from build123d import *

# Parameters (mm, degrees)
F0_W      = 43.942
F0_H      = 2.159
F0_W_2    = 6.858
F1_DEPTH  = 25.4
F0_R      = 2.159
F2_DEPTH  = 3.175
F3_R      = 2.159
F4_DEPTH  = 3.175
F6_R      = 2.159
F7_DEPTH  = 3.175
F9_R      = 2.159
F10_DEPTH = 3.175


with BuildPart() as f1:
    # F0 (on Right) → F1 (new body)
    with BuildSketch(Plane.YZ):
        with Locations((-17.288983049, 3.5224220661)):
            Rectangle(F0_W, F0_H)
        with Locations((8.111016951, 3.5224220661)):
            Rectangle(F0_W_2, F0_H)
    extrude(amount=F1_DEPTH)

    # F0 (on Right) → F2 (join)
    with BuildSketch(Plane.YZ):
        with BuildLine():
            Line((4.682016951, 8.5389220661), (4.682016951, 4.6019220661))
            Line((4.682016951, 4.6019220661), (11.540016951, 4.6019220661))
            Line((11.540016951, 4.6019220661), (11.540016951, 8.5389220661))
            ThreePointArc((11.540016951, 8.5389220661), (8.111016951, 5.1099220661), (4.682016951, 8.5389220661))
        make_face()
        with BuildLine():
            ThreePointArc((11.540016951, 8.5389220661), (8.111016951, 11.9679220661), (4.682016951, 8.5389220661))
            ThreePointArc((4.682016951, 8.5389220661), (8.111016951, 5.1099220661), (11.540016951, 8.5389220661))
        make_face()
        with Locations((8.111016951, 8.5389220661)):
            Circle(F0_R, mode=Mode.SUBTRACT)
    extrude(amount=F2_DEPTH)

    # F3 (on face) → F4 (join)
    with BuildSketch(Plane.YZ.offset(25.4)):
        with BuildLine():
            ThreePointArc((4.682016951, 8.5389220661), (8.111016951, 5.1099220661), (11.540016951, 8.5389220661))
            ThreePointArc((11.540016951, 8.5389220661), (8.111016951, 11.9679220661), (4.682016951, 8.5389220661))
        make_face()
        with Locations((8.111016951, 8.5389220661)):
            Circle(F3_R, mode=Mode.SUBTRACT)
        with BuildLine():
            Line((11.540016951, 4.6019220661), (11.540016951, 8.5389220661))
            ThreePointArc((11.540016951, 8.5389220661), (8.111016951, 5.1099220661), (4.682016951, 8.5389220661))
            Line((4.682016951, 8.5389220661), (4.682016951, 4.6019220661))
            Line((4.682016951, 4.6019220661), (11.540016951, 4.6019220661))
        make_face()
    extrude(amount=-F4_DEPTH)

    # F6 (on offset) → F7 (join)
    with BuildSketch(Plane.YZ.offset(7.112)):
        with BuildLine():
            Line((11.540016951, 4.6019220661), (11.540016951, 8.5389220661))
            ThreePointArc((11.540016951, 8.5389220661), (8.111016951, 11.9679220661), (4.682016951, 8.5389220661))
            Line((4.682016951, 8.5389220661), (4.682016951, 4.6019220661))
            Line((4.682016951, 4.6019220661), (11.540016951, 4.6019220661))
        make_face()
        with Locations((8.111016951, 8.5389220661)):
            Circle(F6_R, mode=Mode.SUBTRACT)
    extrude(amount=F7_DEPTH)

    # F9 (on offset) → F10 (join)
    with BuildSketch(Plane.YZ.offset(18.288)):
        with BuildLine():
            Line((4.682016951, 8.5389220661), (4.682016951, 4.6019220661))
            Line((4.682016951, 4.6019220661), (11.540016951, 4.6019220661))
            Line((11.540016951, 4.6019220661), (11.540016951, 8.5389220661))
            ThreePointArc((11.540016951, 8.5389220661), (8.111016951, 11.9679220661), (4.682016951, 8.5389220661))
        make_face()
        with Locations((8.111016951, 8.5389220661)):
            Circle(F9_R, mode=Mode.SUBTRACT)
    extrude(amount=-F10_DEPTH)


solid = f1.part
Can you work these out from the model? Positions are in its coordinate system, mm. A direction names the side the tool comes from. Round coordinates to 2 decimals unless told otherwise and drop trailing zeros. Write each loop counter-clockwise with the first axis right and the second up, starting at its lowest first coordinate (ties: lowest second). Pieces come first, ordered by that corner, then holes. Notation, with made-up numbers: (20.25, 59.5) -> (52.25, 59.5) arc R29 ccw to (52.25, 89.5) -> close; hole circle Ø7 at (-28, -13). An arc over 180 degrees is marked (long way). One line per question, with ' | ' between items. Start each with the question number.
1) Suppose I cut it at B-B on y = -7. Write out the boundary of the cut face in (x, z).
2) I'm going to push flat-ended pins straight in: P1, Ø1, axis at x = 7.5, z = 9.5, coming from the +Y side; P2, Ø12.5, axis at x = 18.5, y = -22.5, coming from the +Z side; P3, Ø1.6, axis at x = 16, z = 7, coming from the -Y side; P4, Ø3.5, axis at y = 8.11, z = 8.54, coming from the +X side. Where does each tip first touch, or does it pass through?
3) I need wall thicknesses on line 1 (Z direction, x = 22.75, y = -11.5); line 2 (Y direction, x = 1.75, z = 6); line 3 (Y direction, x = 16.5, z = 11.5). Which ranges of each line are inside material? Lowest first, please. Write a range as [from, to].
4) Suppose I cut it at A-A on x = 7.75. Write out the boundary of the cut face in (y, z).
5) On a 3-axis mill with a long thin cutter (end or side, diameter ignored), from which of +Z, -Z, +X, -X, +Y, -Y can I reach the whole of each face in a straight line? I mean faces 1 (the flat face through (24, 4.682, 7)), 2 (the flat face through (3.175, 10, 7)), 3 (the flat face through (25.4, -8, 4)). Say none if no direction works.
6) If we mould it in two halves opening along Y, with no side actions, what happens to faces 4 (the flat face through (9, 4.682, 7)), 5 (the flat face through (10.287, 10, 7)), 6 (the cylindrical face through (23.83, 9.27, 10.36))? For each: released by +Y, released by -Y, zero draft, split by the parting line, or undercut.
7) Suppose I cut it at C-C on x = 21.25. Write out the boundary of the cut face in (y, z), then the cut area to 3 significant figures.
Return value:
1) outline: (0, 2.44) -> (25.4, 2.44) -> (25.4, 4.6) -> (0, 4.6) -> close
2) P1: stops at y = 11.51 | P2: stops at z = 4.6 | P3: stops at y = 4.68 | P4: passes through
3) line 1: z = [2.44, 4.6] | line 2: y = [4.68, 11.54] | line 3: y = [6.38, 9.84]
4) outline: (-39.26, 2.44) -> (11.54, 2.44) -> (11.54, 8.54) arc R3.43 ccw to (4.68, 8.54) -> (4.68, 4.6) -> (-39.26, 4.6) -> close; hole circle Ø4.32 at (8.11, 8.54)
5) face 1: +Z, +X, -X, -Y | face 2: +Z, +Y, -Y | face 3: +Z, -Z, +X, +Y, -Y
6) face 4: released by -Y | face 5: zero draft | face 6: undercut
7) outline: (-39.26, 2.44) -> (11.54, 2.44) -> (11.54, 4.6) -> (-39.26, 4.6) -> close | area: 110 mm2
